from build123d import *

# Parameters (mm, degrees)
BOSS_EXTRUDE1_DEPTH = 304.8
SKETCH2_R           = 10.998522628
BOSS_EXTRUDE2_DEPTH = 12.7
SKETCH3_R           = 44.45
BOSS_EXTRUDE3_DEPTH = 12.7
SKETCH4_W           = 6.35
SKETCH4_H           = 6.35
BOSS_EXTRUDE4_DEPTH = 5.08


with BuildPart() as part:
    # Sketch1 → Boss-Extrude1 (new body)
    with BuildSketch(Plane.XY):
        Polygon((5.499261314, 9.525), (-5.499261314, 9.525), (-10.998522628, 0), (-5.499261314, -9.525), (5.499261314, -9.525), (10.998522628, 0), align=None)
    extrude(amount=BOSS_EXTRUDE1_DEPTH)

    # Sketch2 → Boss-Extrude2 (add)
    with BuildSketch(Plane(origin=(0, 0, 0), x_dir=(-1, 0, 0), z_dir=(0, 0, -1))):
        Circle(SKETCH2_R)
    extrude(amount=-BOSS_EXTRUDE2_DEPTH)

    # Sketch3 → Boss-Extrude3 (add)
    with BuildSketch(Plane(origin=(0, 0, 0), x_dir=(-1, 0, 0), z_dir=(0, 0, -1))):
        Circle(SKETCH3_R)
    extrude(amount=BOSS_EXTRUDE3_DEPTH)

    # Sketch4 → Boss-Extrude4 (add)
    with BuildSketch(Plane(origin=(0, 0, -12.7), x_dir=(-1, 0, 0), z_dir=(0, 0, -1))):
        with Locations((0, 38.1)):
            Rectangle(SKETCH4_W, SKETCH4_H)
    extrude(amount=BOSS_EXTRUDE4_DEPTH)


solid = part.part
Work out the finished part from the listing and answer in its coordinate system (mm). A direction names the side the tool comes from. Coordinates: 2 decimals unless noted, no trailing zeros. Write each loop counter-clockwise with the first axis right and the second up, starting at its lowest first coordinate (ties: lowest second). Pieces come first, ordered by that corner, then holes.
1. The part is cut by section A-A, the plane x = 0. Write down the section's boundary in (y, z) (3 decimals).
Results list:
outline: (-44.45, -12.7) - (34.925, -12.7) - (34.925, -17.78) - (41.275, -17.78) - (41.275, -12.7) - (44.45, -12.7) - (44.45, 0) - (10.999, 0) - (10.999, 12.7) - (9.525, 12.7) - (9.525, 304.8) - (-9.525, 304.8) - (-9.525, 12.7) - (-10.999, 12.7) - (-10.999, 0) - (-44.45, 0) - close
2. Flat-ended cylindrical pins translate along their axes: pin 1 (2.5 mm diameter, centred on y = 38.5, z = -15.5, fed in from +X) (3 decimals); pin 2 (5 mm diameter, centred on x = 35.5, y = 27, fed in from -Z); pin 3 (2 mm diameter, centred on y = -8.5, z = 26, fed in from -X). Find the tip coordinate at first contact, or state that the pin passes through.
Results list:
pin 1: stops at x = 3.175
pin 2: stops at z = -12.7
pin 3: stops at x = -6.67
3. The part is cut by section B-B, the plane z = 276. Write down the section's boundary in (x, y) (3 decimals).
Results list:
outline: (-10.999, 0) - (-5.499, -9.525) - (5.499, -9.525) - (10.999, 0) - (5.499, 9.525) - (-5.499, 9.525) - close
4. For faces 1 (the flat face through (0, 9.525, 157)), 2 (the flat face through (-8.287, -4.696, 156.705)), 3 (the flat face through (8.21, -4.83, 156.71)), 4 (the cylindrical face through (2.384, -10.737, 6.261)), 5 (the flat face through (0, -9.525, 157)), determine the directions among +Z, -Z, +X, -X, +Y, -Y from which every point of the face is accessible in a straight line to the end or side of a thin tool.
Results list:
face 1: +Z, +X, -X, +Y
face 2: +Z, -X, -Y
face 3: +Z, +X, -Y
face 4: +Z
face 5: +Z, +X, -X, -Y
5. Consider line 1 along Z through (x, y) = (13.5, 22.5); line 2 along Z through (x, y) = (-5, -3); line 3 along Y through (x, z) = (4, 164.5) (3 decimals). Determine where each line is inside the solid, lowest interval first.
Results list:
line 1: z = -12.7 to 0
line 2: z = -12.7 to 304.8
line 3: y = -9.525 to 9.525
6. The part is cut by section C-C, the plane y = 3. Write down the section's boundary in (x, z), and give its area (3 significant figures).
Results list:
outline: (-44.35, -12.7) - (44.35, -12.7) - (44.35, 0) - (10.58, 0) - (10.58, 12.7) - (9.27, 12.7) - (9.27, 304.8) - (-9.27, 304.8) - (-9.27, 12.7) - (-10.58, 12.7) - (-10.58, 0) - (-44.35, 0) - close
area: 6,810 mm2
7. The part is cut by section D-D, the plane y = -33.5. Write down the section's boundary in (x, z).
Results list:
outline: (-29.22, -12.7) - (29.22, -12.7) - (29.22, 0) - (-29.22, 0) - close
